from build123d import *

# Parameters (mm, degrees)
BOSS_EXTRUDE1_DEPTH = 210.295833
SKETCH3_R           = 77.5
CUT_EXTRUDE1_DEPTH  = 145
SKETCH5_R           = 2.1
SKETCH5_W           = 5
SKETCH5_H           = 20
CUT_EXTRUDE2_DEPTH  = 5
BOSS_EXTRUDE3_DEPTH = 5


with BuildPart() as part:
    # Sketch2 → Boss-Extrude1 (new body)
    with BuildSketch(Plane.XY.offset(2)):
        Polygon((9824.878184466, 584.85282122), (9909.787083107, 615.730562883), (9909.90527281, 610.4531895), (9826.586986711, 580.153885714), align=None)
    extrude(amount=BOSS_EXTRUDE1_DEPTH)

    # Sketch3 → Cut-Extrude1 (cut)
    with BuildSketch(Plane.XY.offset(156.31)):
        with Locations((9942.206448078, 615.592583846)):
            Circle(SKETCH3_R)
    extrude(amount=-CUT_EXTRUDE1_DEPTH, mode=Mode.SUBTRACT)

    # Sketch5 → Cut-Extrude2 (cut)
    with BuildSketch(Plane(origin=(959.703546547, -2639.032739095, 0), x_dir=(0.939787101, 0.341760449, 0), z_dir=(-0.341760449, 0.939787101, 0))):
        with Locations((9435.67335083, -159.721874806)):
            Circle(SKETCH5_R)
        with Locations((9435.67335083, -54.573958269)):
            Circle(SKETCH5_R)
        Polygon((9480.447890116, -212.295833075), (9476.247890116, -212.295833075), (9476.247890116, -208.295833075), (9474.547890116, -208.295833075), (9474.547890116, -205.495833075), (9476.247890116, -205.495833075), (9476.247890116, -195.495833075), (9480.447890116, -195.495833075), (9480.447890116, -205.495833075), (9482.147890116, -205.495833075), (9482.147890116, -208.295833075), (9480.447890116, -208.295833075), align=None)
        with Locations((9435.67335083, -187.058853941)):
            Rectangle(SKETCH5_W, SKETCH5_H)
        with Locations((9435.67335083, -107.147916538)):
            Rectangle(SKETCH5_W, SKETCH5_H)
        with Locations((9435.67335083, -27.236979134)):
            Rectangle(SKETCH5_W, SKETCH5_H)
        Polygon((9453.115424439, -2), (9457.315424439, -2), (9457.315424439, -6), (9459.015424439, -6), (9459.015424439, -8.8), (9457.315424439, -8.8), (9457.315424439, -18.8), (9453.115424439, -18.8), (9453.115424439, -8.8), (9451.415424439, -8.8), (9451.415424439, -6), (9453.115424439, -6), align=None)
    extrude(amount=-CUT_EXTRUDE2_DEPTH, mode=Mode.SUBTRACT)

    # Sketch7 → Boss-Extrude3 (add)
    with BuildSketch(Plane(origin=(959.703546547, -2639.032739095, 0), x_dir=(0.939787101, 0.341760449, 0), z_dir=(-0.341760449, 0.939787101, 0))):
        with BuildLine():
            Line((9433.17335083, -49.573958269), (9433.17335083, -59.573958269))
            ThreePointArc((9433.17335083, -59.573958269), (9430.083180886, -54.573958269), (9433.17335083, -49.573958269))
        make_face()
        with BuildLine():
            Line((9433.17335083, -154.721874806), (9433.17335083, -164.721874806))
            ThreePointArc((9433.17335083, -164.721874806), (9430.083180886, -159.721874806), (9433.17335083, -154.721874806))
        make_face()
    extrude(amount=-BOSS_EXTRUDE3_DEPTH)


solid = part.part
Geometry: final body of the model. Coordinates: model frame, mm. A direction names the side the tool comes from. Round coordinates to 2 decimals unless told otherwise and drop trailing zeros. Loops run counter-clockwise (first coordinate to the right, second up) from the corner with the lowest first, then second, coordinate; pieces in that order, holes last. Notation, with made-up numbers: (-18.75, 12) -> (1.25, 12) arc R14 ccw to (1.25, 19) -> close; hole circle Ø3 at (4, 68.5). An arc over 180 degrees is marked (long way). One line per question, with ' | ' between items. Start each with the question number.
1. Section C-C on z = 34. Output: boundary loops of the cut face in (x, y) (3 decimals).
2. Line query: line 1 along Z through (x, y) = (9886, 604.5); line 2 along Y through (x, z) = (9853, 75); line 3 along Y through (x, z) = (9837, 80.5). Output: solid intervals per line, ascending. Write a range as [from, to].
3. Section A-A on x = 9900. Output: boundary loops of the cut face in (y, z), and give its area (3 significant figures).
4. Contact query for a flat-ended pin moving along its axis: pin 1 (12 mm diameter, centred on x = 9862.5, y = 583, fed in from -Z). Output: stop coordinate, or through.
5. Mould query, pull axis Z, two halves, no side actions, for faces 1 (the face through (9828, 583, 97.148)), 2 (the face through (9866.2, 597.26, 210.32)), 3 (the face through (9888, 605, 11.31)), 4 (the face through (9846, 591, 212.296)). Classes: pulls with the +Z half, pulls with the -Z half, needs draft (parallel to the pull), parting line crosses it, or undercut.
6. Section B-B on y = 607. Output: boundary loops of the cut face in (x, z), and give its area (3 significant figures).
7. Section D-D on x = 9858.5. Output: boundary loops of the cut face in (y, z), and give its area (3 significant figures).
8. Set-up query: faces 5 (the face through (9825.745, 582.47, 135.672)), 6 (the face through (9825.745, 582.47, 204.571)), 7 (the face through (9848.41, 590.79, 13.73)). Return all of +Z, -Z, +X, -X, +Y, -Y with unobstructed straight access to the full face (end or side cutting, diameter ignored); none if empty.
Returned:
1) outline: (9829.577, 586.562) -> (9831.286, 581.863) -> (9867.485, 595.027) arc R77.5 cw to (9866.308, 599.919) -> close
2) line 1: z = [2, 11.31], [156.31, 212.3] | line 2: y = [589.76, 595.08] | line 3: y = [583.94, 589.26]
3) outline: (606.85, 2) -> (612.17, 2) -> (612.17, 11.31) -> (606.85, 11.31) -> close; (606.85, 156.31) -> (612.17, 156.31) -> (612.17, 212.3) -> (606.85, 212.3) -> close | area: 347 mm2
4) pin 1: passes through
5) face 1: undercut | face 2: needs draft | face 3: undercut | face 4: pulls with the +Z half
6) outline: (9885.78, 2) -> (9900.41, 2) -> (9900.41, 11.31) -> (9885.78, 11.31) -> close; (9885.78, 156.31) -> (9900.41, 156.31) -> (9900.41, 212.3) -> (9885.78, 212.3) -> close | area: 955 mm2
7) outline: (591.76, 2) -> (597.08, 2) -> (597.08, 212.3) -> (591.76, 212.3) -> close | area: 1,120 mm2
8) face 5: -X, -Y | face 6: +Z, -X, -Y | face 7: -Z, -Y
